from build123d import *

# Parameters (mm, degrees)
F0_R     = 25
F1_DEPTH = 25
F2_W     = 25
F2_H     = 20
F3_DEPTH = 10
F3_TAPER = 3


with BuildPart() as f1:
    # F0 (on Top) → F1 (new body)
    with BuildSketch(Plane.XY):
        Circle(F0_R)
    extrude(amount=F1_DEPTH)

    # F2 (on face) → F3 (cut)
    with BuildSketch(Plane.XY.offset(25)):
        Rectangle(F2_W, F2_H)
    extrude(amount=-F3_DEPTH, taper=F3_TAPER, mode=Mode.SUBTRACT)


solid = f1.part
Could you check a few things on this model? Use its own coordinates, in mm. Give positions to 0.01 mm unless a question says otherwise; leave off trailing zeros. Order: outer loops, then holes, each group sorted by start corner. A loop starts at its lowest first (then second) coordinate and runs counter-clockwise, first axis right, second up. Notation, with made-up numbers: (18.5, 40) - (73.5, 40) arc R10 ccw to (73.5, 47) - close; hole circle Ø2 at (-9, 35). An arc over 180 degrees is marked (long way). Return JSON: item names as keys, results as strings. Group by question number.
Q1. Suppose I cut it at A-A, the plane z = 7.25. Please give me the cut outline in (x, y), and give its area (3 significant figures).
Q2. Thinking about a two-plate mould opening in Y: for faces 1 (the face through (0, 0, 0)), 2 (the face through (0, 0, 15)), 3 (the face through (23.846, 7.509, 12.325)), which applies, pulls with the +Y half, pulls with the -Y half, needs draft (parallel to the pull), parting line crosses it, or undercut?
Q3. Suppose I cut it at B-B, the plane x = 15. Please give me the cut outline in (y, z).
Q4. Please list where these lines run through material, in increasing order: line 1 along Z through (x, y) = (0.5, 2.5); line 2 along X through (y, z) = (23, 8.25); line 3 along X through (y, z) = (4, 16). Write a range as [from, to].
Q5. Will these pins go through, and if not, where does the flat tip stop? pin 1 Ø3 at (y, z) = (-16, 9) entering from -X; pin 2 Ø12 at (x, y) = (2.5, -17.5) entering from -Z; pin 3 Ø3 at (x, z) = (4, 15) entering from +Y; pin 4 Ø1.5 at (y, z) = (-6.5, 10.5) entering from -X.
Resolved:
{
 "1": {"outline": "circle Ø50 at (0, 0)", "area": "1,960 mm2"},
 "2": {"face 1": "needs draft", "face 2": "undercut", "face 3": "parting line crosses it"},
 "3": {"outline": "(-20, 0) - (20, 0) - (20, 25) - (-20, 25) - close"},
 "4": {"line 1": "z = [0, 15]", "line 2": "x = [-9.8, 9.8]", "line 3": "x = [-24.68, -12.03], [12.03, 24.68]"},
 "5": {"pin 1": "stops at x = -20.37", "pin 2": "stops at z = 0", "pin 3": "stops at y = 24.87", "pin 4": "stops at x = -24.33"}
}
